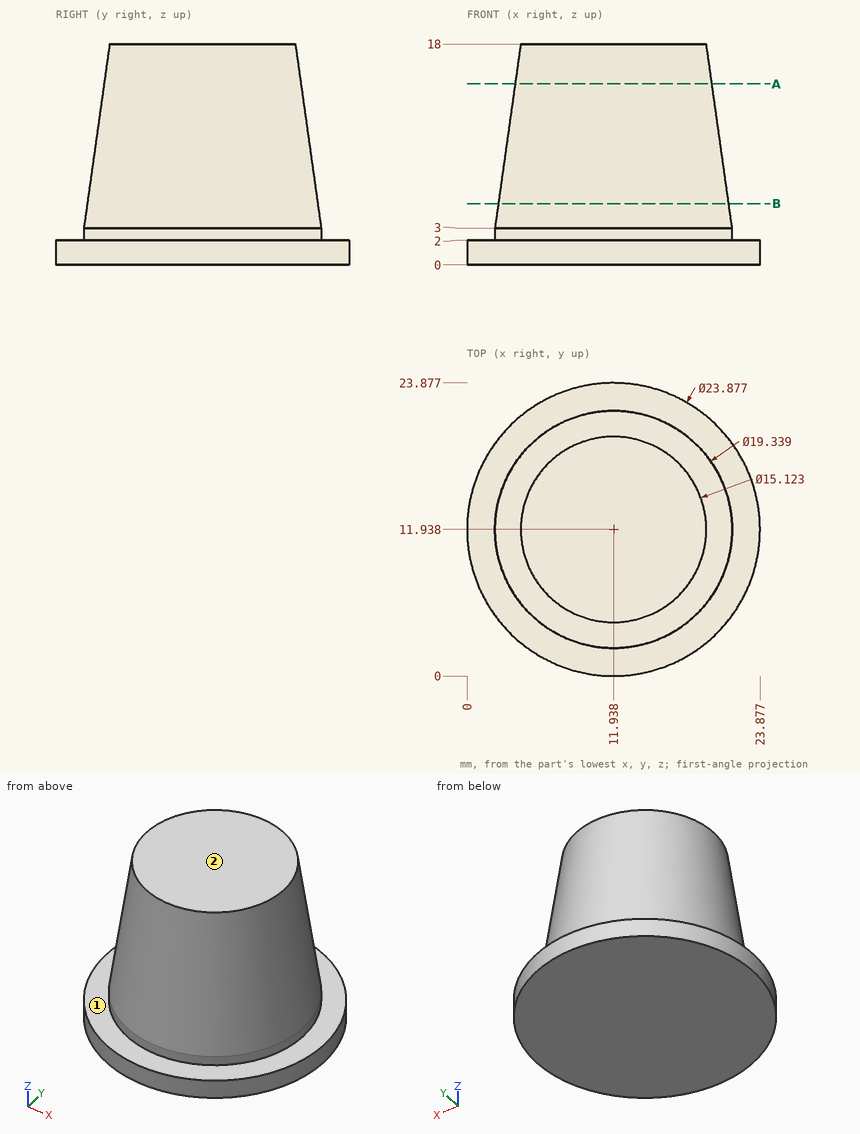
Source: three-view drawing plus pictorial views. Frame: mm from the lowest corner of the part. A direction names the side the tool comes from. Give positions to 0.01 mm unless a question says otherwise; leave off trailing zeros. Loops run counter-clockwise (first coordinate to the right, second up) from the corner with the lowest first, then second, coordinate; pieces in that order, holes last. Notation, with made-up numbers: (47.25, 5) -> (71.25, 5) arc R20 ccw to (71.25, 35) -> close; hole circle Ø7 at (-7, -34.5). An arc over 180 degrees is marked (long way). Put each result on its own line as item: value. Start each with the question number.
1) Reachability of the marked faces 1 and 2 from +Z, -Z, +X, -X, +Y, -Y: full face, straight path, thin tool, end or side. Return the list, or none.
2) Cut plane A-A (z = 14.75). Return loops of the section in (x, y), then the cut area to 3 significant figures.
3) Contact query for flat-ended pins moving along their axis: P1, Ø1.5, axis at y = 20, z = 13.5, coming from the +X side (1 decimal); P2, Ø4, axis at y = 7.5, z = 5.5, coming from the +X side; P3, Ø5, axis at x = 7, z = 14.5, coming from the +Y side. Output: stop coordinate, or through.
4) Cut plane B-B (z = 5). Return loops of the section in (x, y).
5) Material intervals for probe 1 along Z at (x, y) = (2.5, 18); probe 2 along Y at (x, z) = (7.25, 5.5) (1 decimal); probe 3 along X at (y, z) = (12.25, 3.5) (1 decimal), sorted ascending.
Results are:
1. face 1: +Z
1. face 2: +Z, +X, -X, +Y, -Y
2. outline: circle Ø16.04 at (11.94, 11.94)
2. area: 202 mm2
3. P1: stops at x = 15.7
3. P2: stops at x = 21
3. P3: stops at y = 19.69
4. outline: circle Ø18.78 at (11.94, 11.94)
5. probe 1: z = 0 to 2
5. probe 2: y = 3.9 to 20
5. probe 3: x = 2.3 to 21.5
